```python
from build123d import *


with BuildPart() as f1:
    # F0 (on Front) → F1 (revolve)
    with BuildSketch(Plane.XZ):
        Polygon((15.2590650846, 9.8613593727), (16.9848029748, 0), (18, 0), (16.2742621098, 9.8613593727), align=None)
        Polygon((11, 40), (11, 34.1988741416), (15.2590650846, 9.8613593727), (16.2742621098, 9.8613593727), align=None)
        Polygon((9.9848029748, 40), (11, 34.1988741416), (11, 40), align=None)
    revolve(axis=Axis((0, 0, 20), (0, 0, 1)))


solid = f1.part
```
Geometry check sheet. Reference: the model listing, model coordinates, mm. Coordinates: 2 decimals unless noted, no trailing zeros. Write each loop counter-clockwise with the first axis right and the second up, starting at its lowest first coordinate (ties: lowest second). Pieces come first, ordered by that corner, then holes. Notation, with made-up numbers: M 30,10 L 86,10 A17 cw 86,33 Z; hole C 39.25,62.5 d6. An arc over 180 degrees is marked long. Answer as a JSON object with one key per item and string values.
1. Section check A-A, the plane z = 33. Enter the section's corners in (x, y) (3 decimals), plus the area to 3 significant figures.
Answers below:
{"outline": "C 0,0 d24.45; hole C 0,0 d22.42", "area": "74.7 mm²"}
2. Section check B-B, the plane z = 8.5. Enter the section's corners in (x, y) (1 decimal).
Answers below:
{"outline": "C 0,0 d33; hole C 0,0 d31"}
3. Go/stop test with flat-tipped pins: pin 1 Ø5 at (x, y) = (4, -3.5) entering from +Z; pin 2 Ø2 at (y, z) = (9.5, 16) entering from +X; pin 3 Ø4 at (x, z) = (-13.5, 31.5) entering from -Y; pin 4 Ø4 at (x, z) = (7, 33) entering from +Y. Record where each tip stops, or that it passes through.
Answers below:
{"pin 1": "passes through", "pin 2": "stops at x = 12.63", "pin 3": "stops at y = -4.95", "pin 4": "stops at y = 11.23"}
4. Scan lines: L1, parallel to Y at x = -6, z = 5; L2, parallel to X at y = -2, z = 9.5; L3, parallel to Y at x = -11, z = 26. Record each from-to range of solid material in increasing order.
Answers below:
{"L1": "y = -16.04 to -14.95, 14.95 to 16.04", "L2": "x = -16.21 to -15.19, 15.19 to 16.21", "L3": "y = -7.74 to -5.8, 5.8 to 7.74"}
